```python
from build123d import *

# Parameters (mm, degrees)
F0_R     = 5
F0_R_2   = 20
F1_DEPTH = 9


with BuildPart() as f1:
    # F0 (on Front) → F1 (new body)
    with BuildSketch(Plane.XZ):
        Polygon((-78, -52), (-78, -57), (78, -57), (78, -52), (78, 52), (78, 57), (-78, 57), (-78, 52), align=None)
        with Locations((-70, -49)):
            Circle(F0_R, mode=Mode.SUBTRACT)
        with Locations((70, -49)):
            Circle(F0_R, mode=Mode.SUBTRACT)
        with Locations((-70, 49)):
            Circle(F0_R, mode=Mode.SUBTRACT)
        Circle(F0_R_2, mode=Mode.SUBTRACT)
        with Locations((70, 49)):
            Circle(F0_R, mode=Mode.SUBTRACT)
    extrude(amount=F1_DEPTH)


solid = f1.part
```
Check sheet for the modelled part. Datum: model origin and axes. Units: mm. Round coordinates to 2 decimals unless told otherwise and drop trailing zeros. Loops run counter-clockwise (first coordinate to the right, second up) from the corner with the lowest first, then second, coordinate; pieces in that order, holes last. Notation, with made-up numbers: (6, 42.25) - (61, 42.25) arc R16 ccw to (61, 52.25) - close; hole circle Ø7 at (80.25, -7.75). An arc over 180 degrees is marked (long way). Answer as a JSON object with one key per item and string values. Group by question number.
Q1. Scan lines: line 1 along Z through (x, y) = (-70, -4.75); line 2 along X through (y, z) = (-5, -44.5); line 3 along Z through (x, y) = (0, -3.75). Record each from-to range of solid material in increasing order. Write a range as [from, to].
Q2. Sectioned sample at A-A, the plane x = 0. Enter the section's corners in (y, z), plus the area to 3 significant figures.
Q3. Sectioned sample at D-D, the plane y = -6.75. Enter the section's corners in (x, z).
Q4. Sectioned sample at C-C, the plane x = 70. Enter the section's corners in (y, z).
Q5. Gauge pin test, flat ends, axial feed: P1, Ø13, axis at x = 70, z = -49, coming from the -Y side; P2, Ø9, axis at x = 70, z = 49, coming from the +Y side. Record the tip position at first contact, or that the pin passes through.
Q6. Sectioned sample at B-B, the plane z = -49. Enter the section's corners in (x, y), plus the area to 3 significant figures.
Q7. Mould release check, pull along X, two halves, no side actions. Record for faces 1 (the face through (78, -4, -1)), 2 (the face through (73, -4, 53)), 3 (the face through (-4.336, -4.437, -19.524)), 4 (the face through (-78, -4, 1)): released by +X, released by -X, zero draft, split by the parting line, or undercut.
Solution:
{
 "1": {"line 1": "z = [-57, -54], [-44, 44], [54, 57]", "line 2": "x = [-78, -72.18], [-67.82, 67.82], [72.18, 78]", "line 3": "z = [-57, -20], [20, 57]"},
 "2": {"outline": "(-9, -57) - (0, -57) - (0, -20) - (-9, -20) - close; (-9, 20) - (0, 20) - (0, 57) - (-9, 57) - close", "area": "666 mm²"},
 "3": {"outline": "(-78, -57) - (78, -57) - (78, 57) - (-78, 57) - close; hole circle Ø10 at (-70, -49); hole circle Ø10 at (-70, 49); hole circle Ø40 at (0, 0); hole circle Ø10 at (70, -49); hole circle Ø10 at (70, 49)"},
 "4": {"outline": "(-9, -57) - (0, -57) - (0, -54) - (-9, -54) - close; (-9, -44) - (0, -44) - (0, 44) - (-9, 44) - close; (-9, 54) - (0, 54) - (0, 57) - (-9, 57) - close"},
 "5": {"P1": "stops at y = -9", "P2": "passes through"},
 "6": {"outline": "(-78, -9) - (-75, -9) - (-75, 0) - (-78, 0) - close; (-65, -9) - (65, -9) - (65, 0) - (-65, 0) - close; (75, -9) - (78, -9) - (78, 0) - (75, 0) - close", "area": "1,220 mm²"},
 "7": {"face 1": "released by +X", "face 2": "undercut", "face 3": "undercut", "face 4": "released by -X"}
}
